Geometry: final body of the model. Coordinates: model frame, mm. A direction names the side the tool comes from. Give positions to 0.01 mm unless a question says otherwise; leave off trailing zeros. Order: outer loops, then holes, each group sorted by start corner. A loop starts at its lowest first (then second) coordinate and runs counter-clockwise, first axis right, second up. Notation, with made-up numbers: (42.25, -26) - (63.25, -26) arc R13 ccw to (63.25, -10) - close; hole circle Ø8 at (83.25, 18). An arc over 180 degrees is marked (long way). One line per item, written item: value.
```python
from build123d import *

# Parameters (mm, degrees)
F0_W     = 31.5
F0_H     = 11
F1_DEPTH = 79
F2_W     = 28
F2_H     = 8
F2_H_2   = 11
F3_DEPTH = 10


with BuildPart() as f1:
    # F0 (on Front) → F1 (new body)
    with BuildSketch(Plane.XZ):
        Rectangle(F0_W, F0_H)
    extrude(amount=F1_DEPTH)

    # F2 (on face) → F3 (cut)
    with BuildSketch(Plane.XY.offset(5.5)):
        with Locations((0, -6)):
            Rectangle(F2_W, F2_H)
        with Locations((0, -17.5)):
            Rectangle(F2_W, F2_H_2)
        with Locations((0, -30.5)):
            Rectangle(F2_W, F2_H_2)
        with Locations((0, -43.5)):
            Rectangle(F2_W, F2_H_2)
        with Locations((0, -56.5)):
            Rectangle(F2_W, F2_H_2)
        with Locations((0, -69.5)):
            Rectangle(F2_W, F2_H_2)
    extrude(amount=-F3_DEPTH, mode=Mode.SUBTRACT)


solid = f1.part
```
1) Set-up query: faces 4 (the face through (0, -79, 0)), 5 (the face through (0, -43, -4.5)). Return all of +Z, -Z, +X, -X, +Y, -Y with unobstructed straight access to the full face (end or side cutting, diameter ignored); none if empty.
Answers below:
face 4: +Z, -Z, +X, -X, -Y
face 5: +Z
2) First-contact query: pin 1 (3.5 mm diameter, centred on x = 4.5, y = -59, fed in from +Z). Flat tip, straight axial feed; report the tip coordinate or a pass-through.
Answers below:
pin 1: z = -4.5
3) Section A-A, the plane z = -2.5. Return loops of the section in (x, y).
Answers below:
outline: (-15.75, -79) - (15.75, -79) - (15.75, 0) - (-15.75, 0) - close; hole (-14, -75) - (14, -75) - (14, -64) - (-14, -64) - close; hole (-14, -62) - (14, -62) - (14, -51) - (-14, -51) - close; hole (-14, -49) - (14, -49) - (14, -38) - (-14, -38) - close; hole (-14, -36) - (14, -36) - (14, -25) - (-14, -25) - close; hole (-14, -23) - (14, -23) - (14, -12) - (-14, -12) - close; hole (-14, -10) - (14, -10) - (14, -2) - (-14, -2) - close
4) Mould query, pull axis X, two halves, no side actions, for faces 1 (the face through (0, -39, -5.5)), 2 (the face through (-15.75, -39, 0)), 3 (the face through (0, -2, 1)). Classes: released by +X, released by -X, zero draft, split by the parting line, or undercut.
Answers below:
face 1: zero draft
face 2: released by -X
face 3: undercut
5) Section B-B, the plane x = 3. Return loops of the section in (y, z), then the cut area to 3 significant figures.
Answers below:
outline: (-79, -5.5) - (0, -5.5) - (0, 5.5) - (-2, 5.5) - (-2, -4.5) - (-10, -4.5) - (-10, 5.5) - (-12, 5.5) - (-12, -4.5) - (-23, -4.5) - (-23, 5.5) - (-25, 5.5) - (-25, -4.5) - (-36, -4.5) - (-36, 5.5) - (-38, 5.5) - (-38, -4.5) - (-49, -4.5) - (-49, 5.5) - (-51, 5.5) - (-51, -4.5) - (-62, -4.5) - (-62, 5.5) - (-64, 5.5) - (-64, -4.5) - (-75, -4.5) - (-75, 5.5) - (-79, 5.5) - close
area: 239 mm^2
6) Material intervals for line 1 along X through (y, z) = (-57.5, 5); line 2 along Z through (x, y) = (5, -15), sorted ascending.
Answers below:
line 1: -15.75 to -14, 14 to 15.75
line 2: -5.5 to -4.5
7) Section C-C, the plane y = -13. Return loops of the section in (x, z), then the cut area to 3 significant figures.
Answers below:
outline: (-15.75, -5.5) - (15.75, -5.5) - (15.75, 5.5) - (14, 5.5) - (14, -4.5) - (-14, -4.5) - (-14, 5.5) - (-15.75, 5.5) - close
area: 66.5 mm^2
